```python
from build123d import *

# Parameters (mm, degrees)
SKETCH_1_R      = 2
SKETCH_1_R_2    = 1.55
SKETCH_1_W      = 6.1
SKETCH_1_H      = 10
EXTRUDE_1_DEPTH = 6


with BuildPart() as part:
    # Эскиз1 → Бобышка-Вытянуть1 (new body)
    with BuildSketch(Plane(origin=(0, 0, 0), x_dir=(1, 0, 0), z_dir=(0, 1, 0))):
        with BuildLine():
            Line((-121.241078921, -80.805954046), (-129.241078921, -88.805954046))
            Line((-129.241078921, -88.805954046), (-129.241078921, -99.805954046))
            ThreePointArc((-129.241078921, -99.805954046), (-128.069506046, -102.634381171), (-125.241078921, -103.805954046))
            Line((-125.241078921, -103.805954046), (86.758921079, -103.805954046))
            ThreePointArc((86.758921079, -103.805954046), (89.587348204, -102.634381171), (90.758921079, -99.805954046))
            Line((90.758921079, -99.805954046), (90.758921079, -88.805954046))
            Line((90.758921079, -88.805954046), (82.758921079, -80.805954046))
            Line((82.758921079, -80.805954046), (82.758921079, 93.194045954))
            Line((82.758921079, 93.194045954), (90.758921079, 101.194045954))
            Line((90.758921079, 101.194045954), (90.758921079, 112.194045954))
            ThreePointArc((90.758921079, 112.194045954), (89.587348204, 115.022473079), (86.758921079, 116.194045954))
            Line((86.758921079, 116.194045954), (-125.241078921, 116.194045954))
            ThreePointArc((-125.241078921, 116.194045954), (-128.069506046, 115.022473079), (-129.241078921, 112.194045954))
            Line((-129.241078921, 112.194045954), (-129.241078921, 101.194045954))
            Line((-129.241078921, 101.194045954), (-121.241078921, 93.194045954))
            Line((-121.241078921, 93.194045954), (-121.241078921, -80.805954046))
        make_face()
        with Locations((-123.441078921, -98.305954046)):
            Circle(SKETCH_1_R, mode=Mode.SUBTRACT)
        with Locations((84.958921079, -98.305954046)):
            Circle(SKETCH_1_R, mode=Mode.SUBTRACT)
        with Locations((-123.441078921, 110.694045954)):
            Circle(SKETCH_1_R, mode=Mode.SUBTRACT)
        with Locations((84.958921079, 110.694045954)):
            Circle(SKETCH_1_R, mode=Mode.SUBTRACT)
        with Locations((64.308921079, 86.194045954)):
            Circle(SKETCH_1_R_2, mode=Mode.SUBTRACT)
        with Locations((64.308921079, -73.805954046)):
            Circle(SKETCH_1_R_2, mode=Mode.SUBTRACT)
        with Locations((-102.791078921, -73.805954046)):
            Circle(SKETCH_1_R_2, mode=Mode.SUBTRACT)
        with Locations((-102.791078921, 86.194045954)):
            Circle(SKETCH_1_R_2, mode=Mode.SUBTRACT)
        with Locations((-102.791078921, 61.194045954)):
            Rectangle(SKETCH_1_W, SKETCH_1_H, mode=Mode.SUBTRACT)
        with Locations((64.308921079, -48.805954046)):
            Rectangle(SKETCH_1_W, SKETCH_1_H, mode=Mode.SUBTRACT)
        with BuildLine():
            Line((-59.241078921, -72.747079543), (20.758921079, -72.747079543))
            ThreePointArc((20.758921079, -72.747079543), (25.378318741, -69.660496705), (24.294454985, -64.211545637))
            Line((24.294454985, -64.211545637), (-15.705545015, -24.211545637))
            ThreePointArc((-15.705545015, -24.211545637), (-19.241078921, -22.747079543), (-22.776612827, -24.211545637))
            Line((-22.776612827, -24.211545637), (-62.776612827, -64.211545637))
            ThreePointArc((-62.776612827, -64.211545637), (-63.860476584, -69.660496705), (-59.241078921, -72.747079543))
        make_face(mode=Mode.SUBTRACT)
        with Locations((64.308921079, 61.194045954)):
            Rectangle(SKETCH_1_W, SKETCH_1_H, mode=Mode.SUBTRACT)
        with BuildLine():
            Line((20.758921079, 85.135171451), (-59.241078921, 85.135171451))
            ThreePointArc((-59.241078921, 85.135171451), (-63.860476584, 82.048588613), (-62.776612827, 76.599637545))
            Line((-62.776612827, 76.599637545), (-22.776612827, 36.599637545))
            ThreePointArc((-22.776612827, 36.599637545), (-19.241078921, 35.135171451), (-15.705545015, 36.599637545))
            Line((-15.705545015, 36.599637545), (24.294454985, 76.599637545))
            ThreePointArc((24.294454985, 76.599637545), (25.378318741, 82.048588613), (20.758921079, 85.135171451))
        make_face(mode=Mode.SUBTRACT)
        with BuildLine():
            Line((59.700046576, -33.805954046), (59.700046576, 46.194045954))
            ThreePointArc((59.700046576, 46.194045954), (56.613463738, 50.813443617), (51.16451267, 49.72957986))
            Line((51.16451267, 49.72957986), (11.16451267, 9.72957986))
            ThreePointArc((11.16451267, 9.72957986), (9.700046576, 6.194045954), (11.16451267, 2.658512048))
            Line((11.16451267, 2.658512048), (51.16451267, -37.341487952))
            ThreePointArc((51.16451267, -37.341487952), (56.613463738, -38.425351709), (59.700046576, -33.805954046))
        make_face(mode=Mode.SUBTRACT)
        with BuildLine():
            Line((-98.182204418, 46.194045954), (-98.182204418, -33.805954046))
            ThreePointArc((-98.182204418, -33.805954046), (-95.09562158, -38.425351709), (-89.646670512, -37.341487952))
            Line((-89.646670512, -37.341487952), (-49.646670512, 2.658512048))
            ThreePointArc((-49.646670512, 2.658512048), (-48.182204418, 6.194045954), (-49.646670512, 9.72957986))
            Line((-49.646670512, 9.72957986), (-89.646670512, 49.72957986))
            ThreePointArc((-89.646670512, 49.72957986), (-95.09562158, 50.813443617), (-98.182204418, 46.194045954))
        make_face(mode=Mode.SUBTRACT)
        with Locations((-102.791078921, -48.805954046)):
            Rectangle(SKETCH_1_W, SKETCH_1_H, mode=Mode.SUBTRACT)
    extrude(amount=EXTRUDE_1_DEPTH)


solid = part.part
```
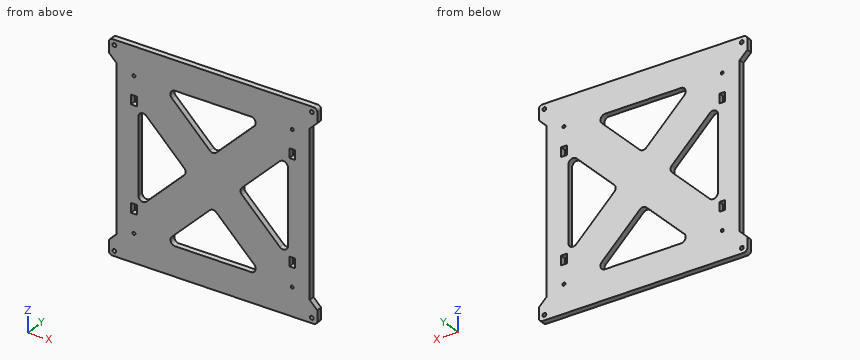
Geometry check sheet. Reference: the model listing, model coordinates, mm. Give positions to 0.01 mm unless a question says otherwise; leave off trailing zeros. Order: outer loops, then holes, each group sorted by start corner. A loop starts at its lowest first (then second) coordinate and runs counter-clockwise, first axis right, second up. Notation, with made-up numbers: (54.5, 9.25) - (102.5, 9.25) arc R28 ccw to (102.5, 32.25) - close; hole circle Ø6 at (85.5, -33.75). An arc over 180 degrees is marked (long way). Answer in a Markdown table with one row per item. Add a question column.
Q1. Cross-section at A-A, the plane z = 1.5. Enter the section's corners in (x, y).
Q2. Material ranges on probe 1 along X at (y, z) = (0.4, 74); probe 2 along Z at (x, y) = (-20, 3.4); probe 3 along Z at (x, y) = (-101, 3.2), recorded low to high. Write a range as from..to.
Q3. Cross-section at D-D, the plane z = 27. Enter the section's corners in (x, y).
Q4. Gauge pin test, flat ends, axial feed: pin 1 (1.8 mm diameter, centred on y = 1.5, z = 50, fed in from -X); pin 2 (3.5 mm diameter, centred on x = 84.96, z = -110.69, fed in from -Y); pin 3 (1.5 mm diameter, centred on y = 3.5, z = 25, fed in from +X). Record the tip position at first contact, or that the pin passes through.
Q5. Cross-section at C-C, the plane z = -81.5. Enter the section's corners in (x, y), then the cut area to 3 significant figures.
Q6. Cross-section at B-B, the plane x = -31.5. Enter the section's corners in (y, z), then the cut area to 3 significant figures.
Check values:
| question | item | result |
|---|---|---|
| 1 | outline | (-121.24, 0) - (-98.18, 0) - (-98.18, 6) - (-121.24, 6) - close; (-53.81, 0) - (15.32, 0) - (15.32, 6) - (-53.81, 6) - close; (59.7, 0) - (82.76, 0) - (82.76, 6) - (59.7, 6) - close |
| 2 | probe 1 | x = -121.24..-104.33, -101.25..62.77, 65.85..82.76 |
| 2 | probe 2 | z = -116.19..-85.14, -35.19..22.81, 72.75..103.81 |
| 2 | probe 3 | z = -116.19..-66.19, -56.19..43.81, 53.81..103.81 |
| 3 | outline | (-121.24, 0) - (-98.18, 0) - (-98.18, 6) - (-121.24, 6) - close; (-79.31, 0) - (-25.57, 0) - (-25.57, 6) - (-79.31, 6) - close; (-12.92, 0) - (40.82, 0) - (40.82, 6) - (-12.92, 6) - close; (59.7, 0) - (82.76, 0) - (82.76, 6) - (59.7, 6) - close |
| 4 | pin 1 | stops at x = -121.24 |
| 4 | pin 2 | passes through |
| 4 | pin 3 | stops at x = 82.76 |
| 5 | outline | (-121.24, 0) - (-64.05, 0) - (-64.05, 6) - (-121.24, 6) - close; (25.57, 0) - (82.76, 0) - (82.76, 6) - (25.57, 6) - close |
| 5 | area | 686 mm^2 |
| 6 | outline | (0, -116.19) - (6, -116.19) - (6, -85.14) - (0, -85.14) - close; (0, -45.32) - (6, -45.32) - (6, 32.93) - (0, 32.93) - close; (0, 72.75) - (6, 72.75) - (6, 103.81) - (0, 103.81) - close |
| 6 | area | 842 mm^2 |
